from build123d import *

# Parameters (mm, degrees)
BOSS_EXTRUDE1_DEPTH = 4
SKETCH2_R           = 23
BOSS_EXTRUDE2_DEPTH = 4
SKETCH3_R           = 45
BOSS_EXTRUDE3_DEPTH = 6
SKETCH4_R           = 40
SKETCH4_R_2         = 19
CUT_EXTRUDE1_DEPTH  = 6
SKETCH5_R           = 14
CUT_EXTRUDE2_DEPTH  = 8
SKETCH6_R           = 7
CUT_EXTRUDE3_DEPTH  = 7
FILLET1_R           = 2
SKETCH7_R           = 3.5
CUT_EXTRUDE4_DEPTH  = 11


with BuildPart() as part:
    # Sketch1 → Boss-Extrude1 (new body)
    with BuildSketch(Plane(origin=(0, 0, 0), x_dir=(1, 0, 0), z_dir=(0, 1, 0))):
        with BuildLine():
            Line((-2, 60.044427996), (-51, 31.754264805))
            ThreePointArc((-51, 31.754264805), (-52.464101615, 30.29016319), (-53, 28.29016319))
            Line((-53, 28.29016319), (-53, -28.29016319))
            ThreePointArc((-53, -28.29016319), (-52.464101615, -30.29016319), (-51, -31.754264805))
            Line((-51, -31.754264805), (-2, -60.044427996))
            ThreePointArc((-2, -60.044427996), (0, -60.580326381), (2, -60.044427996))
            Line((2, -60.044427996), (51, -31.754264805))
            ThreePointArc((51, -31.754264805), (52.464101615, -30.29016319), (53, -28.29016319))
            Line((53, -28.29016319), (53, 28.29016319))
            ThreePointArc((53, 28.29016319), (52.464101615, 30.29016319), (51, 31.754264805))
            Line((51, 31.754264805), (2, 60.044427996))
            ThreePointArc((2, 60.044427996), (0, 60.580326381), (-2, 60.044427996))
        make_face()
    extrude(amount=BOSS_EXTRUDE1_DEPTH)

    # Sketch2 → Boss-Extrude2 (add)
    with BuildSketch(Plane(origin=(0, 4, 0), x_dir=(1, 0, 0), z_dir=(0, 1, 0))):
        Circle(SKETCH2_R)
    extrude(amount=BOSS_EXTRUDE2_DEPTH)

    # Sketch3 → Boss-Extrude3 (add)
    with BuildSketch(Plane.XZ):
        Circle(SKETCH3_R)
    extrude(amount=BOSS_EXTRUDE3_DEPTH)

    # Sketch4 → Cut-Extrude1 (cut)
    with BuildSketch(Plane.XZ.offset(6)):
        Circle(SKETCH4_R)
        Circle(SKETCH4_R_2, mode=Mode.SUBTRACT)
    extrude(amount=-CUT_EXTRUDE1_DEPTH, mode=Mode.SUBTRACT)

    # Sketch5 → Cut-Extrude2 (cut)
    with BuildSketch(Plane.XZ.offset(6)):
        Circle(SKETCH5_R)
    extrude(amount=-CUT_EXTRUDE2_DEPTH, mode=Mode.SUBTRACT)

    # Sketch6 → Cut-Extrude3 (cut, through all)
    with BuildSketch(Plane.XZ.offset(-2)):
        Circle(SKETCH6_R)
    extrude(amount=-CUT_EXTRUDE3_DEPTH, mode=Mode.SUBTRACT)

    # Fillet1
    fillet1_edges = [part.edges().sort_by_distance(p)[0] for p in [
        (-23, 4, 0),
        (-45, -6, 0),
        (-19, -6, 0),
    ]]
    fillet(fillet1_edges, radius=FILLET1_R)

    # Sketch7 → Cut-Extrude4 (cut, through all)
    with BuildSketch(Plane(origin=(0, 4, 0), x_dir=(1, 0, 0), z_dir=(0, 1, 0))):
        with Locations((0, 51)):
            Circle(SKETCH7_R)
        with Locations((44.167295593, 25.5)):
            Circle(SKETCH7_R)
        with Locations((44.167295593, -25.5)):
            Circle(SKETCH7_R)
        with Locations((0, -51)):
            Circle(SKETCH7_R)
        with Locations((-44.167295593, -25.5)):
            Circle(SKETCH7_R)
        with Locations((-44.167295593, 25.5)):
            Circle(SKETCH7_R)
    extrude(amount=-CUT_EXTRUDE4_DEPTH, mode=Mode.SUBTRACT)


solid = part.part
Build history of the part. All positions in model axes, mm. A direction names the side the tool comes from. Give positions to 0.01 mm unless a question says otherwise; leave off trailing zeros. Order: outer loops, then holes, each group sorted by start corner. A loop starts at its lowest first (then second) coordinate and runs counter-clockwise, first axis right, second up. Notation, with made-up numbers: M 51,-0.75 L 88,-0.75 A30 cw 88,38.25 Z; hole C 66.25,88.25 d9. An arc over 180 degrees is marked long. Put each result on its own line as item: value.
Item 1: Drop flat-ended pins along their axis: pin 1 Ø9 at (x, z) = (44.17, -25.5) entering from -Y; pin 2 Ø18 at (x, z) = (0, 0) entering from -Y; pin 3 Ø2 at (y, z) = (4, -41.5) entering from +X. Give the stop position or say it passes through.
Results are:
pin 1: y = 0
pin 2: y = 2
pin 3: x = 35.85
Item 2: Which spindle directions (+Z, -Z, +X, -X, +Y, -Y) get a long thin tool onto all of the face, cutting with end or side? Do faces 4 (the face through (-24, 4, 13)), 5 (the face through (20.765, -1.972, -39.923)), 6 (the face through (13, -6, -38)). Say none if no direction does.
Results are:
face 4: +Y
face 5: -Y
face 6: +Z, -Z, +X, -X, -Y
Item 3: Pull direction Z, two halves, no side cores. Call faces 1 (the face through (-8.67, -3.04, -39.05)), 2 (the face through (52.449, 1.972, 30.316)), 3 (the face through (26.843, 1.972, -45.701)): +Z half, -Z half, draft (parallel to the pull), parting line (faces both ways), or undercut.
Results are:
face 1: undercut
face 2: +Z half
face 3: -Z half
Item 4: Cut at B-B on x = 0. Count the separate pieces of the cut face and the enclosed holes in it, then the cut area to 3 significant figures.
Results are:
separate pieces: 4
enclosed holes: 0
area: 591 mm2
Item 5: Wall check: probe 1 along Z at (x, y) = (0, -1.35); probe 2 along Z at (x, y) = (0, 1.5); probe 3 along Z at (x, y) = (16, -4). Give the ranges that are in metal, low to high.
Results are:
probe 1: -45 to -40, -19 to -14, 14 to 19, 40 to 45
probe 2: -60.58 to -54.5, -47.5 to -14, 14 to 47.5, 54.5 to 60.58
probe 3: -42.06 to -36.66, -10.25 to 10.25, 36.66 to 42.06
Item 6: Cut at C-C on z = 51. Write the cut outline in (x, y), then the cut area to 3 significant figures.
Results are:
outline: M -17.67,0 L -3.5,0 L -3.5,4 L -17.67,4 Z; M 3.5,0 L 17.67,0 L 17.67,4 L 3.5,4 Z
area: 113 mm2
